```python
from build123d import *

# Parameters (mm, degrees)
CROQUIS1_W              = 40
CROQUIS1_H              = 50
SALIENTE_EXTRUIR1_DEPTH = 20
CROQUIS2_R              = 12.5
CORTAR_EXTRUIR1_DEPTH   = 51
CROQUIS3_R              = 1.75
CORTAR_EXTRUIR2_DEPTH   = 21
CORTAR_EXTRUIR3_DEPTH   = 41
CROQUIS5_W              = 3.750800051
CROQUIS5_H              = 3
SALIENTE_EXTRUIR3_DEPTH = 3
CORTAR_EXTRUIR5_DEPTH   = 24
CORTAR_EXTRUIR6_DEPTH   = 12
CROQUIS8_W              = 40
CROQUIS8_H              = 50
CORTAR_EXTRUIR7_DEPTH   = 5


with BuildPart() as part:
    # Croquis1 → Saliente-Extruir1 (new body)
    with BuildSketch(Plane(origin=(0, 0, 0), x_dir=(1, 0, 0), z_dir=(0, 1, 0))):
        with Locations((20, 25)):
            Rectangle(CROQUIS1_W, CROQUIS1_H)
    extrude(amount=SALIENTE_EXTRUIR1_DEPTH)

    # Croquis2 → Cortar-Extruir1 (cut, through all)
    with BuildSketch(Plane.XY):
        with Locations((20, 20.2)):
            Circle(CROQUIS2_R)
    extrude(amount=-CORTAR_EXTRUIR1_DEPTH, mode=Mode.SUBTRACT)

    # Croquis3 → Cortar-Extruir2 (cut, through all)
    with BuildSketch(Plane(origin=(0, 20, 0), x_dir=(1, 0, 0), z_dir=(0, 1, 0))):
        with Locations((3.75, 45)):
            Circle(CROQUIS3_R)
        with Locations((36.25, 45)):
            Circle(CROQUIS3_R)
        with Locations((36.25, 5)):
            Circle(CROQUIS3_R)
        with Locations((3.75, 5)):
            Circle(CROQUIS3_R)
    extrude(amount=-CORTAR_EXTRUIR2_DEPTH, mode=Mode.SUBTRACT)

    # Croquis4 → Cortar-Extruir3 (cut, through all)
    with BuildSketch(Plane(origin=(40, 0, 0), x_dir=(0, 0, -1), z_dir=(1, 0, 0))):
        Polygon((25, 20), (37, 20), (37, 8), (13, 8), (13, 20), align=None)
    extrude(amount=-CORTAR_EXTRUIR3_DEPTH, mode=Mode.SUBTRACT)

    # Croquis5 → Saliente-Extruir3 (add)
    with BuildSketch(Plane(origin=(0, 20, 0), x_dir=(1, 0, 0), z_dir=(0, 1, 0))):
        with Locations((5.626200076, 38.5)):
            Rectangle(CROQUIS5_W, CROQUIS5_H)
        with Locations((34.373799924, 11.5)):
            Rectangle(CROQUIS5_W, CROQUIS5_H)
        with Locations((34.373799924, 38.5)):
            Rectangle(CROQUIS5_W, CROQUIS5_H)
        with Locations((5.626200076, 11.5)):
            Rectangle(CROQUIS5_W, CROQUIS5_H)
    extrude(amount=SALIENTE_EXTRUIR3_DEPTH)

    # Croquis6 → Cortar-Extruir5 (cut, through all)
    with BuildSketch(Plane.XZ):
        with BuildLine():
            Line((13.188139939, -19.615331161), (14.501537669, -18.279657152))
            Line((14.501537669, -18.279657152), (16.224863288, -19.28260268))
            ThreePointArc((16.224863288, -19.28260268), (16.575067996, -19.380217097), (16.928320792, -19.294284721))
            ThreePointArc((16.928320792, -19.294284721), (17.469957789, -19.034324312), (18.033343063, -18.825644933))
            ThreePointArc((18.033343063, -18.825644933), (18.340671144, -18.631425053), (18.513928995, -18.31181024))
            Line((18.513928995, -18.31181024), (18.990823409, -16.375751708))
            Line((18.990823409, -16.375751708), (20.864, -16.36))
            Line((20.864, -16.36), (21.373385647, -18.287764816))
            ThreePointArc((21.373385647, -18.287764816), (21.551993955, -18.604420755), (21.862544768, -18.793444837))
            ThreePointArc((21.862544768, -18.793444837), (22.429359729, -18.992620263), (22.975291881, -19.243435206))
            ThreePointArc((22.975291881, -19.243435206), (23.329939845, -19.323414782), (23.678453448, -19.219924782))
            Line((23.678453448, -19.219924782), (25.384668839, -18.188139939))
            Line((25.384668839, -18.188139939), (26.720342848, -19.501537669))
            Line((26.720342848, -19.501537669), (25.71739732, -21.224863288))
            ThreePointArc((25.71739732, -21.224863288), (25.619782903, -21.575067996), (25.705715279, -21.928320792))
            ThreePointArc((25.705715279, -21.928320792), (25.965675688, -22.469957789), (26.174355067, -23.033343063))
            ThreePointArc((26.174355067, -23.033343063), (26.368574947, -23.340671144), (26.68818976, -23.513928995))
            Line((26.68818976, -23.513928995), (28.624248292, -23.990823409))
            Line((28.624248292, -23.990823409), (28.64, -25.864))
            Line((28.64, -25.864), (26.712235184, -26.373385647))
            ThreePointArc((26.712235184, -26.373385647), (26.395579245, -26.551993955), (26.206555163, -26.862544768))
            ThreePointArc((26.206555163, -26.862544768), (26.007379737, -27.429359729), (25.756564794, -27.975291881))
            ThreePointArc((25.756564794, -27.975291881), (25.676585218, -28.329939845), (25.780075218, -28.678453448))
            Line((25.780075218, -28.678453448), (26.811860061, -30.384668839))
            Line((26.811860061, -30.384668839), (25.498462331, -31.720342848))
            Line((25.498462331, -31.720342848), (23.775136712, -30.71739732))
            ThreePointArc((23.775136712, -30.71739732), (23.424932004, -30.619782903), (23.071679208, -30.705715279))
            ThreePointArc((23.071679208, -30.705715279), (22.530042211, -30.965675688), (21.966656937, -31.174355067))
            ThreePointArc((21.966656937, -31.174355067), (21.659328856, -31.368574947), (21.486071005, -31.68818976))
            Line((21.486071005, -31.68818976), (21.009176591, -33.624248292))
            Line((21.009176591, -33.624248292), (19.136, -33.64))
            Line((19.136, -33.64), (18.626614353, -31.712235184))
            ThreePointArc((18.626614353, -31.712235184), (18.448006045, -31.395579245), (18.137455232, -31.206555163))
            ThreePointArc((18.137455232, -31.206555163), (17.570640271, -31.007379737), (17.024708119, -30.756564794))
            ThreePointArc((17.024708119, -30.756564794), (16.670060155, -30.676585218), (16.321546552, -30.780075218))
            Line((16.321546552, -30.780075218), (14.615331161, -31.811860061))
            Line((14.615331161, -31.811860061), (13.279657152, -30.498462331))
            Line((13.279657152, -30.498462331), (14.28260268, -28.775136712))
            ThreePointArc((14.28260268, -28.775136712), (14.380217097, -28.424932004), (14.294284721, -28.071679208))
            ThreePointArc((14.294284721, -28.071679208), (14.208247472, -27.906200724), (14.127008205, -27.738314697))
            ThreePointArc((14.127008205, -27.738314697), (14.125953752, -27.626452127), (14.209575503, -27.552143653))
            Line((14.209575503, -27.552143653), (17.384042323, -26.571445385))
            ThreePointArc((17.384042323, -26.571445385), (23.05159058, -25.021681648), (17.406635637, -23.391542216))
            Line((17.406635637, -23.391542216), (14.170602247, -22.54767412))
            ThreePointArc((14.170602247, -22.54767412), (14.082937198, -22.475491969), (14.08129489, -22.361945826))
            ThreePointArc((14.08129489, -22.361945826), (14.159930296, -22.19215637), (14.243435206, -22.024708119))
            ThreePointArc((14.243435206, -22.024708119), (14.323414782, -21.670060155), (14.219924782, -21.321546552))
            Line((14.219924782, -21.321546552), (13.188139939, -19.615331161))
        make_face()
    extrude(amount=-CORTAR_EXTRUIR5_DEPTH, mode=Mode.SUBTRACT)

    # Croquis7 → Cortar-Extruir6 (cut)
    with BuildSketch(Plane.XZ):
        with BuildLine():
            Line((7.25, -5), (7.25, 0))
            Line((7.25, 0), (0, 0))
            Line((0, 0), (0, -8.5))
            Line((0, -8.5), (3.75, -8.5))
            ThreePointArc((3.75, -8.5), (6.224873734, -7.474873734), (7.25, -5))
        make_face()
        with BuildLine():
            Line((32.75, -5), (32.75, 0))
            Line((32.75, 0), (40, 0))
            Line((40, 0), (40, -8.5))
            Line((40, -8.5), (36.25, -8.5))
            ThreePointArc((36.25, -8.5), (33.775126266, -7.474873734), (32.75, -5))
        make_face()
        with BuildLine():
            Line((36.25, -41.5), (40, -41.5))
            Line((40, -41.5), (40, -50))
            Line((40, -50), (32.75, -50))
            Line((32.75, -50), (32.75, -45))
            ThreePointArc((32.75, -45), (33.775126266, -42.525126266), (36.25, -41.5))
        make_face()
        with BuildLine():
            Line((7.25, -45), (7.25, -50))
            Line((7.25, -50), (0, -50))
            Line((0, -50), (0, -41.5))
            Line((0, -41.5), (3.75, -41.5))
            ThreePointArc((3.75, -41.5), (6.224873734, -42.525126266), (7.25, -45))
        make_face()
    extrude(amount=-CORTAR_EXTRUIR6_DEPTH, mode=Mode.SUBTRACT)

    # Croquis8 → Cortar-Extruir7 (cut)
    with BuildSketch(Plane.XZ):
        with Locations((20, -25)):
            Rectangle(CROQUIS8_W, CROQUIS8_H)
    extrude(amount=-CORTAR_EXTRUIR7_DEPTH, mode=Mode.SUBTRACT)


solid = part.part
```
CAD build for the part. Positions are in the model's coordinates, mm. A direction names the side the tool comes from. Coordinates: 2 decimals unless noted, no trailing zeros. Write each loop counter-clockwise with the first axis right and the second up, starting at its lowest first coordinate (ties: lowest second). Pieces come first, ordered by that corner, then holes. Notation, with made-up numbers: (67.5, 37.5) -> (121.5, 37.5) arc R22 ccw to (121.5, 49.5) -> close; hole circle Ø1 at (4.25, 47). An arc over 180 degrees is marked (long way). Return JSON: item names as keys, results as strings. Group by question number.
Q1. Cut at B-B, the plane x = 20. Give the cut face in (y, z).
Q2. Cut at C-C, the plane x = 10. Give the cut face in (y, z).
Q3. Cut at A-A, the plane y = 21. Give the cut face in (x, z).
Q4. Which spindle directions (+Z, -Z, +X, -X, +Y, -Y) get a long thin tool onto all of the face, cutting with end or side? Do faces 1 (the face through (38, 8, -41.5)), 2 (the face through (38, 8, -8.5)), 3 (the face through (27.69, 6.479, -26.115)), 4 (the face through (3.751, 21, -38)). Say none if no direction does.
Q5. Pull direction X, two halves, no side cores. Call faces 5 (the face through (17.58, 6.48, -31.01)), 6 (the face through (40, 7, -25)), 7 (the face through (37, 12, -47)): released by +X, released by -X, zero draft, split by the parting line, or undercut.
Q6. Drill centre lines: line 1 (Z direction, x = 36.25, y = 17.5); line 2 (X direction, y = 18, z = -5); line 3 (Z direction, x = 35, y = 12.75). Where is each one in solid material? Low to high.
Q7. Flat gauge pins, fed straight in: pin 1 (4 mm diameter, centred on y = 8.5, z = -2, fed in from +X); pin 2 (2 mm diameter, centred on x = 2.5, z = -47, fed in from -Y); pin 3 (14 mm diameter, centred on x = 8.5, z = -25, fed in from +Y). Where does each tip first touch, or does it go through?
Returned:
{
 "1": {"outline": "(5, -50) -> (7.7, -50) -> (7.7, -33.63) -> (5, -33.63) -> close; (5, -28.05) -> (7.7, -28.05) -> (7.7, -21.95) -> (5, -21.95) -> close; (5, -16.37) -> (7.7, -16.37) -> (7.7, 0) -> (5, 0) -> close"},
 "2": {"outline": "(5, -50) -> (12.7, -50) -> (12.7, -37) -> (8, -37) -> (8, -13) -> (12.7, -13) -> (12.7, 0) -> (5, 0) -> close"},
 "3": {"outline": "(3.75, -40) -> (7.5, -40) -> (7.5, -37) -> (3.75, -37) -> close; (3.75, -13) -> (7.5, -13) -> (7.5, -10) -> (3.75, -10) -> close; (32.5, -40) -> (36.25, -40) -> (36.25, -37) -> (32.5, -37) -> close; (32.5, -13) -> (36.25, -13) -> (36.25, -10) -> (32.5, -10) -> close"},
 "4": {"face 1": "-Z, +X, -Y", "face 2": "+Z, +X, -Y", "face 3": "+Y, -Y", "face 4": "+Z, -Z, -X, +Y"},
 "5": {"face 5": "undercut", "face 6": "released by +X", "face 7": "zero draft"},
 "6": {"line 1": "z = -50 to -46.75, -43.25 to -37, -13 to -6.75, -3.25 to 0", "line 2": "x = 0 to 2, 5.5 to 7.7, 32.3 to 34.5, 38 to 40", "line 3": "z = -50 to -46.22, -43.78 to -37, -13 to -6.22, -3.78 to 0"},
 "7": {"pin 1": "stops at x = 32.75", "pin 2": "stops at y = 12", "pin 3": "stops at y = 8"}
}
